```python
from build123d import *

# Parameters (mm, degrees)
F0_R      = 3.75
F1_DEPTH  = 2
F2_R      = 1
F3_DEPTH  = 3
F4_W      = 37.5
F4_H      = 18
F5_DEPTH  = 6
F7_DEPTH  = 18
F8_R      = 2
F9_DEPTH  = 37.8
F10_R     = 0.99999
F11_SIZE  = 5
F12_DEPTH = 14.9


# Not quite as in the source:
# - a fillet or chamfer is up to 0.001 mm smaller than in the source, because OpenCascade refuses the exact size


with BuildPart() as f1:
    # F0 (on Top) → F1 (new body)
    with BuildSketch(Plane.XY):
        Circle(F0_R)
    extrude(amount=F1_DEPTH)

    # F2 (on face) → F3 (join)
    with BuildSketch(Plane.XY.offset(2)):
        Circle(F2_R)
    extrude(amount=F3_DEPTH)

    # F4 (on face) → F5 (join)
    with BuildSketch(Plane.XY.offset(5)):
        with BuildLine():
            Line((22.5, 9), (0, 9))
            Line((0, 9), (0, 1))
            ThreePointArc((0, 1), (0.7071067812, 0.7071067812), (1, 0))
            ThreePointArc((1, 0), (0.7071067812, -0.7071067812), (0, -1))
            Line((0, -1), (0, -9))
            Line((0, -9), (22.5, -9))
            Line((22.5, -9), (22.5, 9))
        make_face()
        with BuildLine():
            ThreePointArc((1, 0), (0.7071067812, 0.7071067812), (0, 1))
            Line((0, 1), (0, -1))
            ThreePointArc((0, -1), (0.7071067812, -0.7071067812), (1, 0))
        make_face()
        with BuildLine():
            Line((0, -1), (0, 1))
            ThreePointArc((0, 1), (-1, 0), (0, -1))
        make_face()
        with BuildLine():
            Line((0, 9), (-6, 9))
            Line((-6, 9), (-6, -9))
            Line((-6, -9), (0, -9))
            Line((0, -9), (0, -1))
            ThreePointArc((0, -1), (-1, 0), (0, 1))
            Line((0, 1), (0, 9))
        make_face()
        with Locations((41.25, 0)):
            Rectangle(F4_W, F4_H)
    extrude(amount=F5_DEPTH)

    # F6 (on face) → F7 (join)
    with BuildSketch(Plane.XZ.offset(9)):
        Polygon((64.2426406871, 9.2426406871), (60, 5), (81.2132034356, -16.2132034356), (85.4558441227, -11.9705627485), align=None)
        Polygon((60, 11), (60, 5), (64.2426406871, 9.2426406871), align=None)
    extrude(amount=-F7_DEPTH)

    # F8 (on face) → F9 (cut)
    with BuildSketch(Plane(origin=(32.5, 0, 32.5), x_dir=(0, -1, 0), z_dir=(-0.7071067812, 0, -0.7071067812))):
        with Locations((0, -53.0515164137)):
            Circle(F8_R)
    extrude(amount=-F9_DEPTH, mode=Mode.SUBTRACT)

    # F10 (radius 1 in the source; OpenCascade refuses exactly that, so slightly less here)
    f10_edges = [f1.edges().sort_by_distance(p)[0] for p in [
        (-3.75, 0, 0),
        (-3.75, 0, 2),
    ]]
    fillet(f10_edges, radius=F10_R)

    # F11
    f11_edges = [f1.edges().sort_by_distance(p)[0] for p in [
        (-6, -9, 8),
        (-6, 9, 8),
        (83.334524, 9, -14.091883),
        (83.334524, -9, -14.091883),
    ]]
    chamfer(f11_edges, length=F11_SIZE)

    # F12 (add): a face of the model
    f12_faces = [f1.faces().sort_by_distance(p)[0] for p in [
        (27.6735454285, 0, 11),
    ]]
    extrude(f12_faces, amount=F12_DEPTH)


solid = f1.part
```
The listing builds one solid part. Answer for the finished solid, in the listing's coordinates (mm). A direction names the side the tool comes from. Round coordinates to 2 decimals unless told otherwise and drop trailing zeros. Order: outer loops, then holes, each group sorted by start corner. A loop starts at its lowest first (then second) coordinate and runs counter-clockwise, first axis right, second up. Notation, with made-up numbers: (9, 50) - (62, 50) arc R5 cw to (62, 59) - close; hole circle Ø4 at (89, 82.5). An arc over 180 degrees is marked (long way). Put each result on its own line as item: value. Start each with the question number.
(1) Find section D-D (z = -10.5). Give the vertices of the cut face in (x, y).
(2) Determine the mould class of faces 5 (the flat face through (81.562, -6.465, -12.379)), 6 (the flat face through (-4, -6, 15)), 7 (the cylindrical face through (70.7, 0.26, -1.52)), 8 (the cylindrical face through (0, -1, 3)) for opening direction Z: released by +Z, released by -Z, zero draft, split by the parting line, or undercut.
(3) Find section C-C (y = 5.5). Give the vertices of the cut face in (x, z), plus the area to 3 significant figures.
(4) For faces 1 (the flat face through (1.2, 0, 2)), 2 (the flat face through (0, 0, 0)), 3 (the flat face through (60, 0, 18)), 4 (the flat face through (31, -9, 15)), determine the directions among +Z, -Z, +X, -X, +Y, -Y from which every point of the face is accessible in a straight line to the end or side of a thin tool.
(5) Given P1, Ø5, axis at y = 3, z = 13, coming from the +X side; P2, Ø2, axis at y = -4, z = 1.5, coming from the -X side; P3, Ø1, axis at x = 50.5, y = -3, coming from the -Z side; P4, Ø3, axis at x = 71, z = 6.5, coming from the -Y side, each flat-ended and moving along its own axis, determine where each tip first touches the part or whether it passes through.
(6) Straight lines are drawn through the part: probe 1 along Z at (x, y) = (22, -5.5); probe 2 along X at (y, z) = (-2.75, 12); probe 3 along X at (y, z) = (-1.25, -12). For each, find the intervals that lie inside material, in ascending order. Write a range as from..to.
Reply:
1. outline: (75.5, -9) - (79.86, -9) - (83.99, -6.08) - (83.99, 6.08) - (79.86, 9) - (75.5, 9) - close
2. face 5: released by -Z
2. face 6: zero draft
2. face 7: undercut
2. face 8: undercut
3. outline: (-4.5, 5) - (60, 5) - (80.15, -15.15) - (84.4, -10.91) - (64.24, 9.24) - (60, 11) - (60, 25.9) - (-4.5, 25.9) - close
3. area: 1,530 mm^2
4. face 1: none
4. face 2: -Z, -X, +Y, -Y
4. face 3: +Z, +X, +Y, -Y
4. face 4: +Z, -Z, +X, -X, -Y
5. P1: x = 61.21
5. P2: x = -2.15
5. P3: z = 5
5. P4: through
6. probe 1: 5..25.9
6. probe 2: -6..60
6. probe 3: 77..85.43
